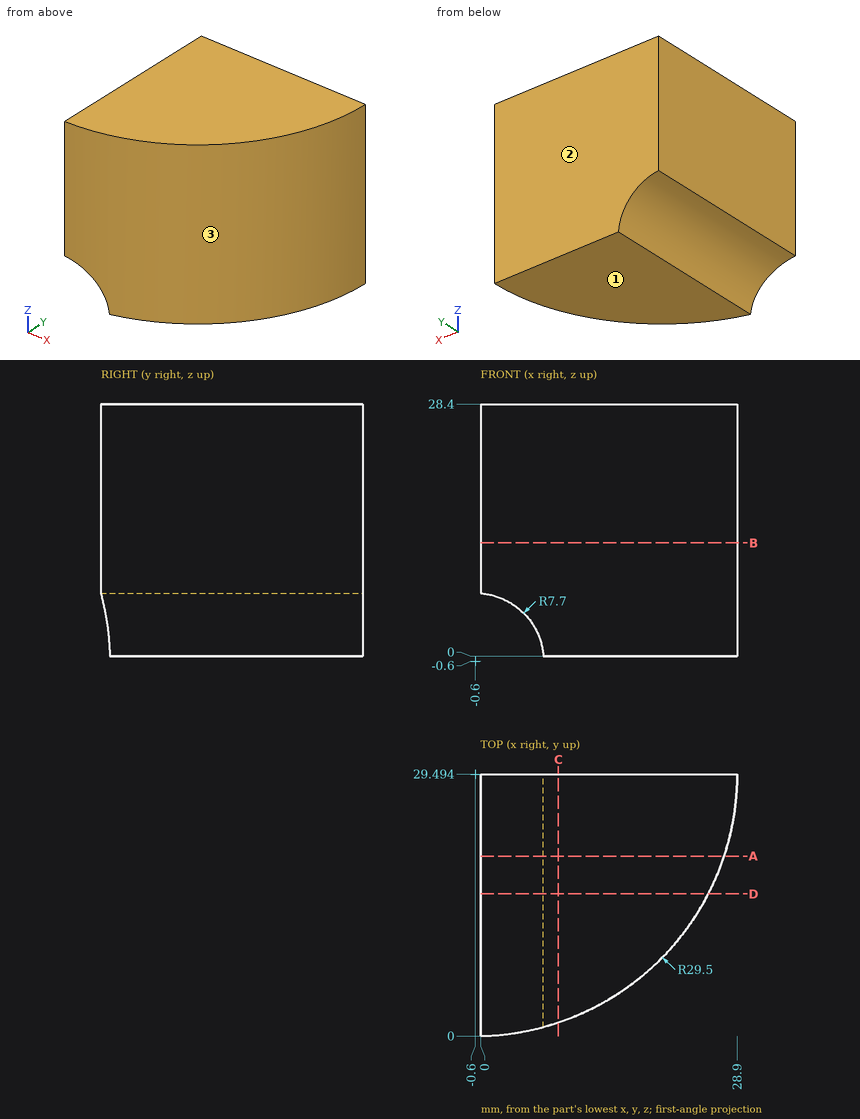
Job drawing, mm, ordinate dimensions from the low corner. One solid piece. Give positions to 0.01 mm unless a question says otherwise; leave off trailing zeros. Loops run counter-clockwise (first coordinate to the right, second up) from the corner with the lowest first, then second, coordinate; pieces in that order, holes last. Notation, with made-up numbers: M 78.5,23.25 L 114.5,23.25 A24 cw 114.5,61.25 Z; hole C -4,78 d9. An arc over 180 degrees is marked long. Return JSON: item names as keys, results as strings.
1) Flat gauge pins, fed straight in: pin 1 Ø8 at (y, z) = (7, 6.5) entering from +X; pin 2 Ø12 at (x, z) = (25, 7.5) entering from -Y; pin 3 Ø12 at (y, z) = (11.5, 4) entering from +X. Where does each tip first touch, or does it go through?
Calculated:
{"pin 1": "stops at x = 22.38", "pin 2": "stops at y = 7.45", "pin 3": "stops at x = 26.35"}
2) Drill centre lines: line 1 (Z direction, x = 3, y = 5); line 2 (X direction, y = 24, z = 1.5); line 3 (X direction, y = 28, z = 5.5). Where is each one in solid material? Low to high.
Calculated:
{"line 1": "z = 6.21 to 28.4", "line 2": "x = 6.81 to 28.38", "line 3": "x = 4.1 to 28.86"}
3) Saw through at B-B, the plane z = 12.75. List the corners of the cut face in (x, y).
Calculated:
{"outline": "M 0,0 A29.5 ccw 28.9,29.49 L 0,29.49 Z"}
4) Saw through at D-D, the plane y = 16. List the corners of the cut face in (x, z).
Calculated:
{"outline": "M 0,7.08 A7.7 cw 7.08,0 L 25.63,0 L 25.63,28.4 L 0,28.4 Z"}
5) Saw through at C-C, the plane x = 8.75. List the corners of the cut face in (y, z) (3 decimals).
Calculated:
{"outline": "M 1.515,0 L 29.494,0 L 29.494,28.4 L 1.515,28.4 Z"}
6) Pull direction Y, two halves, no side cores. Call the marked faces 1, 2 and 3: released by +Y, released by -Y, zero draft, split by the parting line, or undercut.
Calculated:
{"face 1": "zero draft", "face 2": "released by +Y", "face 3": "released by -Y"}
7) Saw through at A-A, the plane y = 20.25. List the corners of the cut face in (x, z).
Calculated:
{"outline": "M 0,7.08 A7.7 cw 7.08,0 L 27.41,0 L 27.41,28.4 L 0,28.4 Z"}
